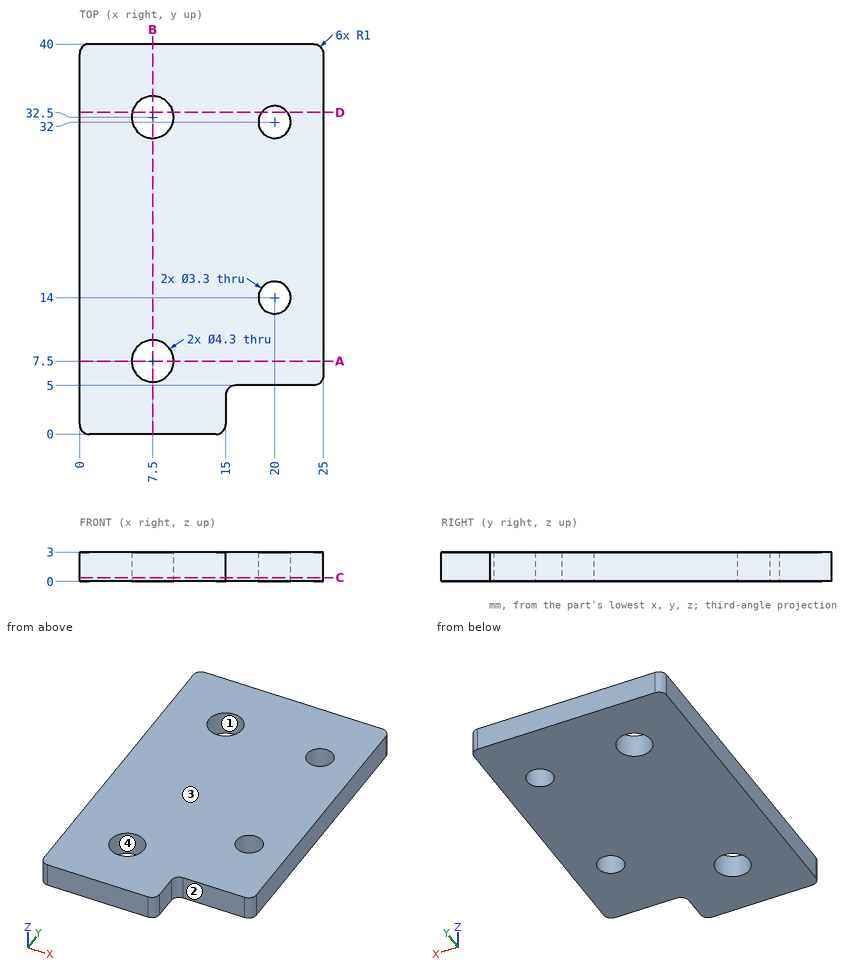
Verification items for this drawing (mm, ordinates from the low corner). A direction names the side the tool comes from. Coordinates: 2 decimals unless noted, no trailing zeros. Order: outer loops, then holes, each group sorted by start corner. A loop starts at its lowest first (then second) coordinate and runs counter-clockwise, first axis right, second up. Notation, with made-up numbers: (6.25, 7.25) -> (17.25, 7.25) arc R32 cw to (17.25, 38.25) -> close; hole circle Ø1 at (59.25, -19.75). An arc over 180 degrees is marked (long way). Put each result on its own line as item: value. Start each with the question number.
1. Material ranges on L1, parallel to Y at x = 20, z = 1.3; L2, parallel to Y at x = 7.5, z = 1.05; L3, parallel to Y at x = 23.25, z = 1.6, recorded low to high. Write a range as [from, to].
2. Go/stop test with flat-tipped pins: pin 1 Ø0.9 at (y, z) = (3, 1) entering from +X; pin 2 Ø0.9 at (x, z) = (22, 2) entering from -Y. Record where each tip stops, or that it passes through.
3. Access from +Z, -Z, +X, -X, +Y, -Y to the whole of each face (thin tool, end or side, straight path). Record for the marked faces 1 and 2.
4. Mould release check, pull along X, two halves, no side actions. Record for the marked faces 3 and 4: released by +X, released by -X, zero draft, split by the parting line, or undercut.
5. Cross-section at C-C, the plane z = 0.4. Record the boundary of the cut face in (x, y).
6. Cross-section at A-A, the plane y = 7.5. Record the boundary of the cut face in (x, z), then the cut area to 3 significant figures.
7. Cross-section at D-D, the plane y = 33. Record the boundary of the cut face in (x, z), then the cut area to 3 significant figures.
8. Cross-section at B-B, the plane x = 7.5. Record the boundary of the cut face in (y, z).
Computed:
1. L1: [5, 12.35], [15.65, 30.35], [33.65, 40]
1. L2: [0, 5.35], [9.65, 30.35], [34.65, 40]
1. L3: [5, 40]
2. pin 1: x = 15
2. pin 2: y = 5
3. face 1: +Z, -Z
3. face 2: +Z, -Z, +X, -Y
4. face 3: zero draft
4. face 4: undercut
5. outline: (0, 1) arc R1 ccw to (1, 0) -> (14, 0) arc R1 ccw to (15, 1) -> (15, 4) arc R1 cw to (16, 5) -> (24, 5) arc R1 ccw to (25, 6) -> (25, 39) arc R1 ccw to (24, 40) -> (1, 40) arc R1 ccw to (0, 39) -> close; hole circle Ø4.3 at (7.5, 7.5); hole circle Ø4.3 at (7.5, 32.5); hole circle Ø3.3 at (20, 14); hole circle Ø3.3 at (20, 32)
6. outline: (0, 0) -> (5.35, 0) -> (5.35, 3) -> (0, 3) -> close; (9.65, 0) -> (25, 0) -> (25, 3) -> (9.65, 3) -> close
6. area: 62.1 mm2
7. outline: (0, 0) -> (5.41, 0) -> (5.41, 3) -> (0, 3) -> close; (9.59, 0) -> (18.69, 0) -> (18.69, 3) -> (9.59, 3) -> close; (21.31, 0) -> (25, 0) -> (25, 3) -> (21.31, 3) -> close
7. area: 54.6 mm2
8. outline: (0, 0) -> (5.35, 0) -> (5.35, 3) -> (0, 3) -> close; (9.65, 0) -> (30.35, 0) -> (30.35, 3) -> (9.65, 3) -> close; (34.65, 0) -> (40, 0) -> (40, 3) -> (34.65, 3) -> close
